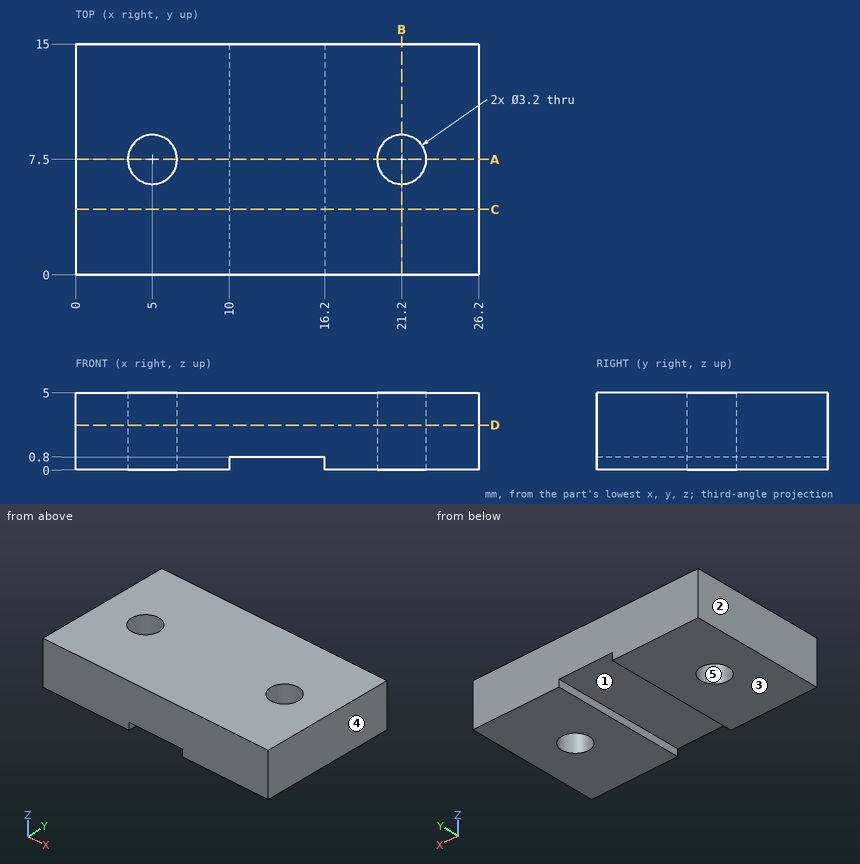
Study the drawing (mm; zero at the part's minimum x, y, z) and answer. A direction names the side the tool comes from. Give positions to 0.01 mm unless a question says otherwise; leave off trailing zeros. Write each loop counter-clockwise with the first axis right and the second up, starting at its lowest first coordinate (ties: lowest second). Pieces come first, ordered by that corner, then holes.
Item 1: Section C-C, the plane y = 4.25 is taken. Write down the section's boundary in (x, z).
Item 2: Section D-D, the plane z = 2.9 is taken. Write down the section's boundary in (x, y).
Item 3: A flat-ended cylindrical pin translates along its axis: P1, Ø2.5, axis at x = 21.2, y = 7.5, coming from the -Z side. Find the tip coordinate at first contact, or state that the pin passes through.
Item 4: Find the intervals of material crossed by line 1 along X through (y, z) = (7.5, 2); line 2 along Y through (x, z) = (5, 2.3); line 3 along X through (y, z) = (6.75, 2.5), in increasing order.
Item 5: Section B-B, the plane x = 21.2 is taken. Write down the section's boundary in (y, z), plus the area to 3 significant figures.
Item 6: Section A-A, the plane y = 7.5 is taken. Write down the section's boundary in (x, z), plus the area to 3 significant figures.
Item 7: Which of the six approach directions +Z, -Z, +X, -X, +Y, -Y give full straight-line access (tool end or side, diameter ignored) to the marked faces 1 and 2?
Item 8: Determine the mould class of the marked faces 3, 4 and 5 for opening direction X: released by +X, released by -X, zero draft, split by the parting line, or undercut.
Completed:
1. outline: (0, 0) - (10, 0) - (10, 0.8) - (16.2, 0.8) - (16.2, 0) - (26.2, 0) - (26.2, 5) - (0, 5) - close
2. outline: (0, 0) - (26.2, 0) - (26.2, 15) - (0, 15) - close; hole circle Ø3.2 at (5, 7.5); hole circle Ø3.2 at (21.2, 7.5)
3. P1: passes through
4. line 1: x = 0 to 3.4, 6.6 to 19.6, 22.8 to 26.2
4. line 2: y = 0 to 5.9, 9.1 to 15
4. line 3: x = 0 to 3.59, 6.41 to 19.79, 22.61 to 26.2
5. outline: (0, 0) - (5.9, 0) - (5.9, 5) - (0, 5) - close; (9.1, 0) - (15, 0) - (15, 5) - (9.1, 5) - close
5. area: 59.0 mm2
6. outline: (0, 0) - (3.4, 0) - (3.4, 5) - (0, 5) - close; (6.6, 0) - (10, 0) - (10, 0.8) - (16.2, 0.8) - (16.2, 0) - (19.6, 0) - (19.6, 5) - (6.6, 5) - close; (22.8, 0) - (26.2, 0) - (26.2, 5) - (22.8, 5) - close
6. area: 94.0 mm2
7. face 1: -Z, +Y, -Y
7. face 2: +Z, -Z, -X, +Y, -Y
8. face 3: zero draft
8. face 4: released by +X
8. face 5: undercut
